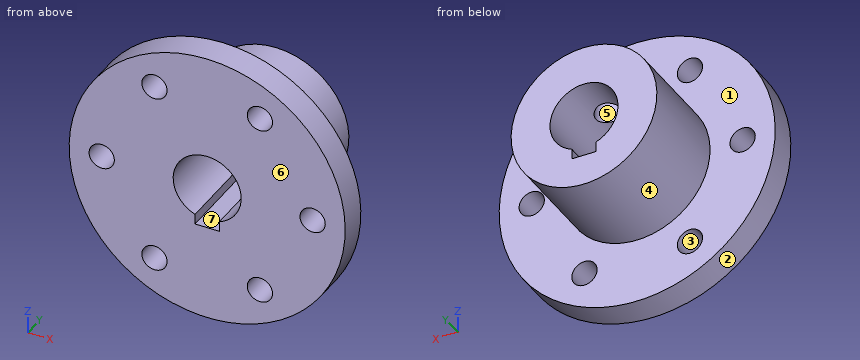
from build123d import *

# Parameters (mm, degrees)
SKETCH1_R           = 28.4
BOSS_EXTRUDE1_DEPTH = 6
SKETCH2_R           = 15
BOSS_EXTRUDE2_DEPTH = 20.4
CUT_EXTRUDE1_DEPTH  = 49.063291606
SKETCH4_R           = 3
CUT_EXTRUDE2_DEPTH  = 49.063291606
SKETCH5_R           = 2.6
CUT_EXTRUDE3_DEPTH  = 46.047530499
CIRPATTERN1_COUNT   = 6


with BuildPart() as part:
    # Sketch1 → Boss-Extrude1 (new body)
    with BuildSketch(Plane(origin=(0, 0, 0), x_dir=(1, 0, 0), z_dir=(0, 1, 0))):
        with Locations(Location((0, 0, 0), (0, 0, 270))):
            Circle(SKETCH1_R)
    extrude(amount=BOSS_EXTRUDE1_DEPTH)

    # Sketch2 → Boss-Extrude2 (add)
    with BuildSketch(Plane(origin=(0, 6, 0), x_dir=(1, 0, 0), z_dir=(0, 1, 0))):
        with Locations(Location((0, 0, 0), (0, 0, 270))):
            Circle(SKETCH2_R)
    extrude(amount=BOSS_EXTRUDE2_DEPTH)

    # Sketch3 → Cut-Extrude1 (cut, through all)
    with BuildSketch(Plane(origin=(0, 26.4, 0), x_dir=(1, 0, 0), z_dir=(0, 1, 0))):
        with BuildLine():
            Line((-2.5, 8.638348415), (2.5, 8.638348415))
            Line((2.5, 8.638348415), (2.5, 6.538348415))
            ThreePointArc((2.5, 6.538348415), (0, -7), (-2.5, 6.538348415))
            Line((-2.5, 6.538348415), (-2.5, 8.638348415))
        make_face()
    extrude(amount=-CUT_EXTRUDE1_DEPTH, mode=Mode.SUBTRACT)

    # Sketch4 → Cut-Extrude2 (cut, through all)
    with BuildSketch(Plane.XY):
        with Locations(Location((0, 16.2, 0), (0, 0, 180))):
            Circle(SKETCH4_R)
    extrude(amount=CUT_EXTRUDE2_DEPTH, mode=Mode.SUBTRACT)

    # Sketch5 → Cut-Extrude3 (cut, through all)
    with BuildSketch(Plane(origin=(0, 6, 0), x_dir=(1, 0, 0), z_dir=(0, 1, 0))):
        with Locations(Location((-21.7, 0, 0), (0, 0, 270))):
            Circle(SKETCH5_R)
    cut_extrude3 = extrude(amount=-CUT_EXTRUDE3_DEPTH, mode=Mode.SUBTRACT)

    # CirPattern1: Cut-Extrude3 ×6 about axis
    cirpattern1_axis = Axis((0, 0, 0), (0, 1, 0))
    for i in range(1, CIRPATTERN1_COUNT):
        add(cut_extrude3.rotate(cirpattern1_axis, i * 360 / CIRPATTERN1_COUNT), mode=Mode.SUBTRACT)


solid = part.part
Verification items for the finished model (mm, model axes). Face numbers are marked on the shaded views. A direction names the side the tool comes from. Give positions to 0.01 mm unless a question says otherwise; leave off trailing zeros. Loops run counter-clockwise (first coordinate to the right, second up) from the corner with the lowest first, then second, coordinate; pieces in that order, holes last.
1) Draft check along X on the marked faces 1, 2 and 3. Enter one of: pulls with the +X half, pulls with the -X half, needs draft (parallel to the pull), parting line crosses it, or undercut.
2) Thickness scan on line 1 along X through (y, z) = (1.9, 0); line 2 along X through (y, z) = (5.75, 19); line 3 along Y through (x, z) = (15, 12). Record the ranges inside material, lowest first.
3) Sectioned sample at C-C, the plane x = 10.5. Enter the section's corners in (y, z), then the cut area to 3 significant figures.
4) Sectioned sample at B-B, the plane x = 22.5. Enter the section's corners in (y, z), then the cut area to 3 significant figures.
5) Set-up check for the marked faces 4, 5, 6 and 7: record each of +Z, -Z, +X, -X, +Y, -Y from which the full face is reachable in a straight line by a thin tool's end or side.
6) Sectioned sample at D-D, the plane z = 11. Enter the section's corners in (x, y).
7) Sectioned sample at A-A, the plane z = 0. Enter the section's corners in (x, y).
8) Depth check by flat-ended pin: pin 1 Ø5 at (x, y) = (0, 16.2) entering from -Z; pin 2 Ø4 at (x, y) = (10.5, 12) entering from -Z; pin 3 Ø1.7 at (y, z) = (10.5, -8) entering from +X. Enter the tip coordinate at first touch or a pass-through.
Answers:
1. face 1: needs draft
1. face 2: parting line crosses it
1. face 3: undercut
2. line 1: x = -28.4 to -24.3, -19.1 to -7, 7 to 19.1, 24.3 to 28.4
2. line 2: x = -21.11 to -13.44, -8.26 to 8.26, 13.44 to 21.11
2. line 3: y = 0 to 6
3. outline: (0, -26.39) - (6, -26.39) - (6, -21.37) - (0, -21.37) - close; (0, -16.22) - (6, -16.22) - (6, -10.71) - (26.4, -10.71) - (26.4, 10.71) - (6, 10.71) - (6, 16.22) - (0, 16.22) - close; (0, 21.37) - (6, 21.37) - (6, 26.39) - (0, 26.39) - close
3. area: 692 mm2
4. outline: (0, -17.33) - (6, -17.33) - (6, -2.47) - (0, -2.47) - close; (0, 2.47) - (6, 2.47) - (6, 17.33) - (0, 17.33) - close
4. area: 178 mm2
5. face 4: +Y
5. face 5: +Z
5. face 6: +Z, -Z, +X, -X, -Y
5. face 7: +Y, -Y
6. outline: (-26.18, 0) - (26.18, 0) - (26.18, 6) - (10.2, 6) - (10.2, 26.4) - (-10.2, 26.4) - (-10.2, 6) - (-26.18, 6) - close; hole circle Ø6 at (0, 16.2)
7. outline: (-28.4, 0) - (-24.3, 0) - (-24.3, 6) - (-28.4, 6) - close; (-19.1, 0) - (-7, 0) - (-7, 26.4) - (-15, 26.4) - (-15, 6) - (-19.1, 6) - close; (7, 0) - (19.1, 0) - (19.1, 6) - (15, 6) - (15, 26.4) - (7, 26.4) - close; (24.3, 0) - (28.4, 0) - (28.4, 6) - (24.3, 6) - close
8. pin 1: stops at z = -15
8. pin 2: stops at z = -12.36
8. pin 3: stops at x = 13.19
